```python
from build123d import *

# Parameters (mm, degrees)
SKETCH1_W           = 40
SKETCH1_H           = 40
BOSS_EXTRUDE1_DEPTH = 40
SKETCH2_W           = 40
SKETCH2_H           = 30
FORK_CUTOUT_DEPTH   = 8
SKETCH5_W           = 3.5
SKETCH5_H           = 11
CUT_EXTRUDE3_DEPTH  = 25
FILLET5_R           = 6
SKETCH6_W           = 1
SKETCH6_H           = 11
CUT_EXTRUDE4_DEPTH  = 6
FILLET6_R           = 2
FILLET8_R           = 2
SKETCH7_W           = 30
SKETCH7_H           = 30
BOSS_EXTRUDE2_DEPTH = 0.1
SKETCH10_W          = 3.75
SKETCH10_H          = 3.75
MARK38_DEPTH        = 0.1
FILLET9_R           = 1


with BuildPart() as part:
    # Sketch1 → Boss-Extrude1 (new body)
    with BuildSketch(Plane(origin=(0, 0, 0), x_dir=(1, 0, 0), z_dir=(0, 1, 0))):
        with Locations((20, 20)):
            Rectangle(SKETCH1_W, SKETCH1_H)
    extrude(amount=BOSS_EXTRUDE1_DEPTH)

    # Sketch2 → Fork Cutout (cut)
    with BuildSketch(Plane.XZ):
        with Locations((20, -20)):
            Rectangle(SKETCH2_W, SKETCH2_H)
    extrude(amount=-FORK_CUTOUT_DEPTH, mode=Mode.SUBTRACT)

    # Sketch5 → Cut-Extrude3 (cut)
    with BuildSketch(Plane(origin=(0, 40, 0), x_dir=(1, 0, 0), z_dir=(0, 1, 0))):
        with Locations((37.25, 20)):
            Rectangle(SKETCH5_W, SKETCH5_H)
    extrude(amount=-CUT_EXTRUDE3_DEPTH, mode=Mode.SUBTRACT)

    # Fillet5
    # the kernel refuses this fillet: 6 mm, written as the material it adds along each edge
    with BuildSketch(Plane(origin=(20.5, 15, -14.5), x_dir=(0, 1, 0), z_dir=(1, 0, 0)), Plane(origin=(39, 15, -25.5), x_dir=(0, 1, 0), z_dir=(-1, 0, 0))) as fillet5_piece_1:
        with BuildLine():
            CenterArc((FILLET5_R, -FILLET5_R), FILLET5_R, 90, 90)
            Line((0, -FILLET5_R), (0, 0))
            Line((0, 0), (FILLET5_R, 0))
        make_face()
    extrude(amount=18.5)

    # Sketch6 → Cut-Extrude4 (cut)
    with BuildSketch(Plane(origin=(0, 40, 0), x_dir=(1, 0, 0), z_dir=(0, 1, 0))):
        with Locations((39.5, 20)):
            Rectangle(SKETCH6_W, SKETCH6_H)
    extrude(amount=-CUT_EXTRUDE4_DEPTH, mode=Mode.SUBTRACT)

    # Fillet6
    fillet6_edges = [part.edges().sort_by_distance(p)[0] for p in [
        (39.5, 34, -25.5),
        (39.5, 34, -14.5),
    ]]
    fillet(fillet6_edges, radius=FILLET6_R)

    # Fillet8
    fillet8_edges = [part.edges().sort_by_distance(p)[0] for p in [
        (20, 8, -5),
        (20, 8, -35),
    ]]
    fillet(fillet8_edges, radius=FILLET8_R)

    # Sketch7 → Boss-Extrude2 (add)
    with BuildSketch(Plane.ZY):
        with Locations((-20, 23.75)):
            Rectangle(SKETCH7_W, SKETCH7_H)
    extrude(amount=BOSS_EXTRUDE2_DEPTH)

    # Sketch10 → Mark38 (cut)
    with BuildSketch(Plane.ZY.offset(0.1)):
        with Locations((-18.125, 33.125)):
            Rectangle(SKETCH10_W, SKETCH10_H)
        Polygon((-20, 27.5), (-12.5, 27.5), (-12.5, 20.128421558), (-16.25, 20.128421558), (-16.25, 16.25), (-20, 16.25), align=None)
        Polygon((-27.5, 35), (-23.75, 35), (-23.75, 16.071209331), (-28.076745998, 16.071209331), (-28.076745998, 12.5), (-31.25, 12.5), (-31.25, 30.980466229), (-27.5, 30.980466229), align=None)
    extrude(amount=-MARK38_DEPTH, mode=Mode.SUBTRACT)

    # Fillet9
    fillet9_edges = [part.edges().sort_by_distance(p)[0] for p in [
        (40, 40, -7.25),
        (20, 40, -40),
        (0, 40, -20),
        (40, 40, -32.75),
        (0, 20, -40),
        (40, 20, -40),
        (40, 20, 0),
        (0, 20, 0),
        (20, 40, 0),
    ]]
    fillet(fillet9_edges, radius=FILLET9_R)


solid = part.part
```
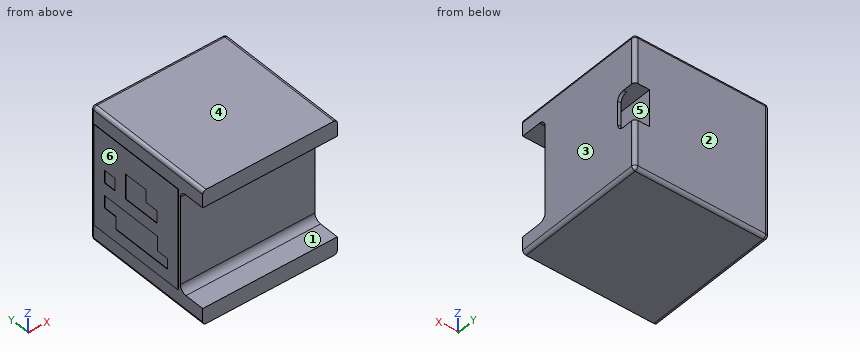
Check sheet for the modelled part. Datum: model origin and axes. Units: mm. Face numbers are marked on the shaded views. A direction names the side the tool comes from. Coordinates: 2 decimals unless noted, no trailing zeros. Order: outer loops, then holes, each group sorted by start corner. A loop starts at its lowest first (then second) coordinate and runs counter-clockwise, first axis right, second up. Notation, with made-up numbers: (-25, 62.5) -> (32, 62.5) arc R24 ccw to (32, 90.5) -> close; hole circle Ø1 at (67, 31.5). An arc over 180 degrees is marked (long way). Write each question's results on one line, items separated by ' | '. Start each with the question number.
1) Section check C-C (x = 37.5). Enter the section's corners in (y, z).
2) Section check A-A (y = 4). Enter the section's corners in (x, z), and give its area (3 significant figures).
3) Set-up check for the marked faces 1 and 2: record each of +Z, -Z, +X, -X, +Y, -Y from which the full face is reachable in a straight line by a thin tool's end or side.
4) Draft check along X on the marked faces 3, 4, 5 and 6. Enter one of: pulls with the +X half, pulls with the -X half, needs draft (parallel to the pull), parting line crosses it, or undercut.
5) Section check D-D (z = -11). Enter the section's corners in (x, y), and give its area (3 significant figures).
6) Section check B-B (y = 24). Enter the section's corners in (x, z).
7) Material ranges on line 1 along X through (y, z) = (23.5, -15); line 2 along X through (y, z) = (33, -16); line 3 along Z through (x, y) = (4.5, 5), recorded low to high.
8) Depth check by flat-ended pin: pin 1 (0.5 mm diameter, centred on x = 39.5, z = -20.5, fed in from +Y); pin 2 (1.9 mm diameter, centred on y = 34, z = -18, fed in from -X). Enter the tip coordinate at first touch or a pass-through.
Checked values:
1) outline: (0, -40) -> (39, -40) arc R1 ccw to (40, -39) -> (40, -25.5) -> (21, -25.5) arc R6 cw to (15.02, -20) arc R6 cw to (21, -14.5) -> (40, -14.5) -> (40, -1) arc R1 ccw to (39, 0) -> (0, 0) -> (0, -5) -> (6, -5) arc R2 cw to (8, -7) -> (8, -33) arc R2 cw to (6, -35) -> (0, -35) -> close
2) outline: (0, -39) arc R1 ccw to (1, -40) -> (39, -40) arc R1 ccw to (40, -39) -> (40, -35) -> (0, -35) -> close; (0, -5) -> (40, -5) -> (40, -1) arc R1 ccw to (39, 0) -> (1, 0) arc R1 ccw to (0, -1) -> close | area: 399 mm²
3) face 1: +X, -X, -Y | face 2: +Z, -Z, +X, -X, +Y
4) face 3: pulls with the +X half | face 4: needs draft | face 5: undercut | face 6: pulls with the -X half
5) outline: (-0.1, 8.75) -> (0, 8.75) -> (0, 8) -> (40, 8) -> (40, 39) arc R1 ccw to (39, 40) -> (1, 40) arc R1 ccw to (0, 39) -> (0, 38.75) -> (-0.1, 38.75) -> close | area: 1,280 mm²
6) outline: (-0.1, -35) -> (0, -35) -> (0, -39) arc R1 ccw to (1, -40) -> (39, -40) arc R1 ccw to (40, -39) -> (40, -1) arc R1 ccw to (39, 0) -> (1, 0) arc R1 ccw to (0, -1) -> (0, -5) -> (-0.1, -5) -> (-0.1, -12.5) -> (0, -12.5) -> (0, -20) -> (-0.1, -20) -> (-0.1, -23.75) -> (0, -23.75) -> (0, -31.25) -> (-0.1, -31.25) -> close; hole (35.5, -25.5) -> (39, -25.5) -> (39, -14.5) -> (35.5, -14.5) -> close
7) line 1: 0 to 35.5, 39 to 40 | line 2: -0.1 to 35.5, 39 to 40 | line 3: -40 to -35, -5 to 0
8) pin 1: y = 34 | pin 2: x = 0
